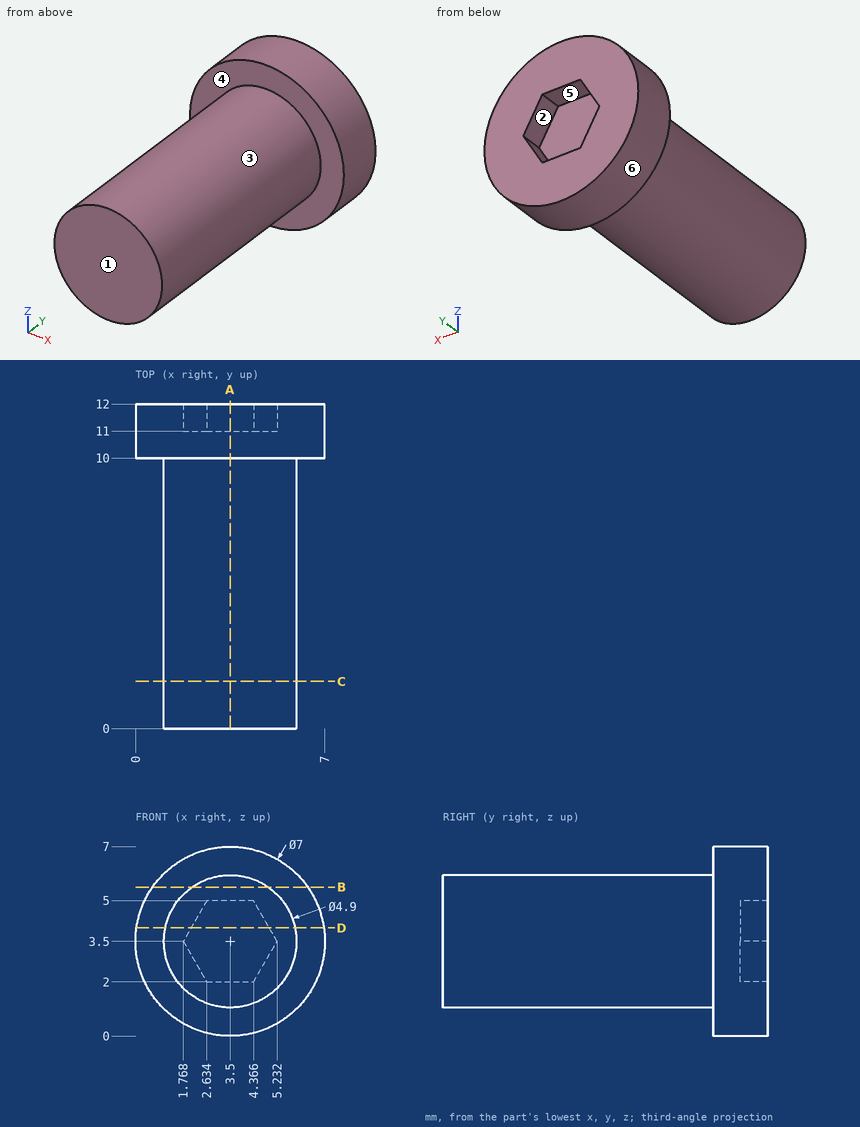
For this review, use the dimensioned drawing (mm, ordinates from the lowest corner) and the shaded views. A direction names the side the tool comes from. Give positions to 0.01 mm unless a question says otherwise; leave off trailing zeros. Loops run counter-clockwise (first coordinate to the right, second up) from the corner with the lowest first, then second, coordinate; pieces in that order, holes last.
Item 1: Tool access review of the marked faces 4, 5 and 6: name each direction out of +Z, -Z, +X, -X, +Y, -Y from which nothing blocks a thin tool from reaching the whole face with its end or side.
Item 2: Take a section at B-B, the plane z = 5.5. State the section outline as (x, y) points (3 decimals).
Item 3: Take a section at C-C, the plane y = 1.75. State the section outline as (x, z) points.
Item 4: For line 1 along Y through (x, z) = (0.75, 5.25); line 2 along Z through (x, y) = (5, 11.75); line 3 along Y through (x, z) = (4.5, 4), list the stretches that pass through material, from the lowest coordinate up.
Item 5: Insertion check: pin 1 (1.5 mm diameter, centred on x = 3, z = 3, fed in from +Y); pin 2 (1 mm diameter, centred on y = 10.5, z = 2.5, fed in from -X); pin 3 (2 mm diameter, centred on x = 2.5, y = 9.5, fed in from -Z). Each pin has a flat end and moves straight along its axis. Give the tip position at first contact, or say it passes through.
Item 6: Take a section at D-D, the plane z = 4. State the section outline as (x, y) points.
Item 7: Draft analysis for pull direction X (two halves, no side actions). For the marked faces 1, 2 and 3, state which applies: +X half, -X half, draft (parallel to the pull), parting line (faces both ways), or undercut.
Item 8: Take a section at A-A, the plane x = 3.5. State the section outline as (y, z) points, and give its area (3 significant figures).
Calculated:
1. face 4: -Y
1. face 5: +Y
1. face 6: +Y, -Y
2. outline: (0.628, 10) - (2.085, 10) - (2.085, 0) - (4.915, 0) - (4.915, 10) - (6.372, 10) - (6.372, 12) - (0.628, 12) - close
3. outline: circle Ø4.9 at (3.5, 3.5)
4. line 1: y = 10 to 12
4. line 2: z = 0.34 to 3.1, 3.9 to 6.66
4. line 3: y = 0 to 11
5. pin 1: stops at y = 11
5. pin 2: stops at x = 0.04
5. pin 3: stops at z = 0
6. outline: (0.04, 10) - (1.1, 10) - (1.1, 0) - (5.9, 0) - (5.9, 10) - (6.96, 10) - (6.96, 12) - (4.94, 12) - (4.94, 11) - (2.06, 11) - (2.06, 12) - (0.04, 12) - close
7. face 1: draft
7. face 2: undercut
7. face 3: parting line
8. outline: (0, 1.05) - (10, 1.05) - (10, 0) - (12, 0) - (12, 2) - (11, 2) - (11, 5) - (12, 5) - (12, 7) - (10, 7) - (10, 5.95) - (0, 5.95) - close
8. area: 60.0 mm2
